Verification items for this drawing (mm, ordinates from the low corner). A direction names the side the tool comes from. Round coordinates to 2 decimals unless told otherwise and drop trailing zeros. Order: outer loops, then holes, each group sorted by start corner. A loop starts at its lowest first (then second) coordinate and runs counter-clockwise, first axis right, second up. Notation, with made-up numbers: (42.25, 24) -> (72.25, 24) arc R20 cw to (72.25, 33) -> close; hole circle Ø8 at (82, 6). An arc over 180 degrees is marked (long way). Return JSON: item names as keys, results as strings. Group by question number.
Item 1: Scan lines: probe 1 along X at (y, z) = (5, 11.1); probe 2 along X at (y, z) = (4.5, 1); probe 3 along Y at (x, z) = (16.5, 10.8). Record each from-to range of solid material in increasing order. Write a range as from..to.
Item 2: Sectioned sample at D-D on z = 10.5. Record the cut outline in (x, y), plus the area to 3 significant figures.
Item 3: Access from +Z, -Z, +X, -X, +Y, -Y to the whole of each face (thin tool, end or side, straight path). Record for the marked faces 4 and 5.
Item 4: Draft check along X on the marked faces 1, 2 and 3. Enter one of: pulls with the +X half, pulls with the -X half, needs draft (parallel to the pull), parting line crosses it, or undercut.
Item 5: Sectioned sample at B-B on y = 5. Record the cut outline in (x, z), plus the area to 3 significant figures.
Item 6: Sectioned sample at A-A on x = 16.5. Record the cut outline in (y, z).
Item 7: Depth check by flat-ended pin: pin 1 Ø3 at (y, z) = (5, 4) entering from -X; pin 2 Ø5 at (x, y) = (8.5, 7) entering from -Z. Enter the tip coordinate at first touch or a pass-through.
Item 8: Sectioned sample at C-C on z = 4. Record the cut outline in (x, y).
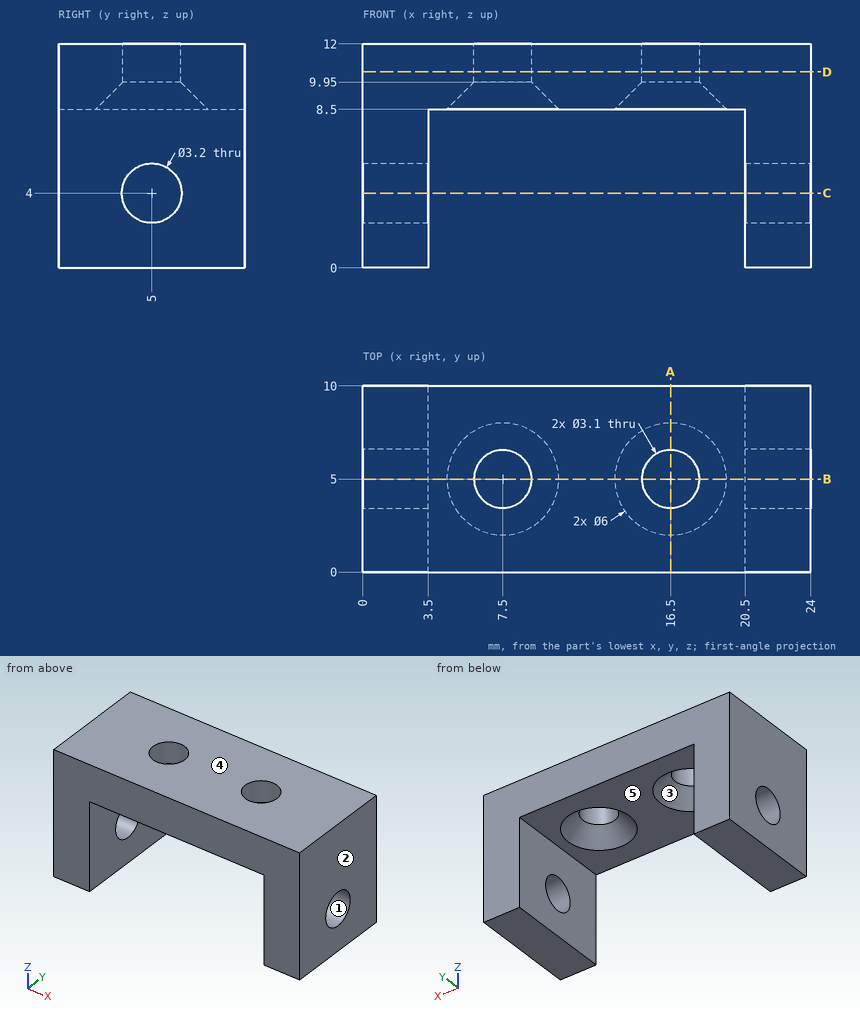
Recorded:
{
 "1": {"probe 1": "0..5.95, 9.05..14.95, 18.05..24", "probe 2": "0..3.5, 20.5..24", "probe 3": "0..3.45, 6.55..10"},
 "2": {"outline": "(0, 0) -> (24, 0) -> (24, 10) -> (0, 10) -> close; hole circle Ø3.1 at (7.5, 5); hole circle Ø3.1 at (16.5, 5)", "area": "225 mm²"},
 "3": {"face 4": "+Z, +X, -X, +Y, -Y", "face 5": "-Z, +Y, -Y"},
 "4": {"face 1": "needs draft", "face 2": "pulls with the +X half", "face 3": "undercut"},
 "5": {"outline": "(0, 0) -> (3.5, 0) -> (3.5, 2.4) -> (0, 2.4) -> close; (0, 5.6) -> (3.5, 5.6) -> (3.5, 8.5) -> (4.5, 8.5) -> (5.95, 9.95) -> (5.95, 12) -> (0, 12) -> close; (9.05, 9.95) -> (10.5, 8.5) -> (13.5, 8.5) -> (14.95, 9.95) -> (14.95, 12) -> (9.05, 12) -> close; (18.05, 9.95) -> (19.5, 8.5) -> (20.5, 8.5) -> (20.5, 5.6) -> (24, 5.6) -> (24, 12) -> (18.05, 12) -> close; (20.5, 0) -> (24, 0) -> (24, 2.4) -> (20.5, 2.4) -> close", "area": "95.2 mm²"},
 "6": {"outline": "(0, 8.5) -> (2, 8.5) -> (3.45, 9.95) -> (3.45, 12) -> (0, 12) -> close; (6.55, 9.95) -> (8, 8.5) -> (10, 8.5) -> (10, 12) -> (6.55, 12) -> close"},
 "7": {"pin 1": "through", "pin 2": "z = 8.5"},
 "8": {"outline": "(0, 0) -> (3.5, 0) -> (3.5, 3.4) -> (0, 3.4) -> close; (0, 6.6) -> (3.5, 6.6) -> (3.5, 10) -> (0, 10) -> close; (20.5, 0) -> (24, 0) -> (24, 3.4) -> (20.5, 3.4) -> close; (20.5, 6.6) -> (24, 6.6) -> (24, 10) -> (20.5, 10) -> close"}
}
